Verification items for the finished model (mm, model axes). A direction names the side the tool comes from. Round coordinates to 2 decimals unless told otherwise and drop trailing zeros. Order: outer loops, then holes, each group sorted by start corner. A loop starts at its lowest first (then second) coordinate and runs counter-clockwise, first axis right, second up. Notation, with made-up numbers: M 52,71.5 L 82,71.5 A29 ccw 82,99.5 Z; hole C 33,8 d10. An arc over 180 degrees is marked long. Use one line per item in the form item = value. Start each with the question number.
Item 1: Thickness scan on probe 1 along Z at (x, y) = (-10, -26.5); probe 2 along X at (y, z) = (-9, -8.5); probe 3 along Z at (x, y) = (49.5, -9). Record the ranges inside material, lowest first. Write a range as [from, to].
Item 2: Release check for a two-part mould opening along X. For faces 1 (the cylindrical face through (15.86, -41.49, 1.72)), 2 (the flat face through (17, -41, -49.969)), 3 (the cylindrical face through (16.509, -11.997, -2.13)) record: +X half, -X half, draft (parallel to the pull), parting line (faces both ways), or undercut.
Item 3: Tool access check on faces 4 (the flat face through (20, -29, -28.969)), 5 (the cylindrical face through (15.93, -38.49, -61.98)), 6 (the flat face through (-9.8, -7.8, -15.969)). Record the directions out of +Z, -Z, +X, -X, +Y, -Y that give a thin tool (end or side, any length) a straight path to the whole face; none if there is none.
Item 4: Go/stop test with flat-tipped pins: pin 1 Ø3 at (y, z) = (-30.5, 32.5) entering from -X; pin 2 Ø2 at (y, z) = (-5, -19.5) entering from +X; pin 3 Ø2 at (x, y) = (47, -4) entering from +Z. Record where each tip stops, or that it passes through.
Item 5: Cross-section at A-A on z = 22.5. Enter the section's corners in (x, y).
from build123d import *

# Parameters (mm, degrees)
F2_W      = 103.9337478578
F2_H      = 131.3569024205
F3_DEPTH  = 50
F4_R      = 8
F5_DEPTH  = 7
F6_R      = 7.5
F7_DEPTH  = 2
F8_R      = 6.5
F9_DEPTH  = 11
F10_R     = 3.5
F11_DEPTH = 11
F12_R     = 1.5
F13_DEPTH = 4
F14_R     = 2.5
F15_DEPTH = 15
F17_START = -4
F16_R     = 6.5
F17_DEPTH = 21.001
F19_DEPTH = 3


with BuildPart() as f1:
    # F0 (on Front) → F1 (revolve)
    with BuildSketch(Plane.XZ):
        with BuildLine():
            Line((58.2725809174, 57.0314990246), (54.7725809174, 57.0314990246))
            Line((54.7725809174, 57.0314990246), (54.7725809174, -8.9685009754))
            Line((54.7725809174, -8.9685009754), (33.7725809174, -8.9685009754))
            Line((33.7725809174, -8.9685009754), (33.7725809174, 2.9023842439))
            Line((33.7725809174, 2.9023842439), (30.7725809174, 4.9023842439))
            Line((30.7725809174, 4.9023842439), (28.7725809174, 4.9023842439))
            Line((28.7725809174, 4.9023842439), (28.7725809174, -8.9685009754))
            Line((28.7725809174, -8.9685009754), (26.7725809174, -8.9685009754))
            Line((26.7725809174, -8.9685009754), (26.7725809174, -10.9685009754))
            Line((26.7725809174, -10.9685009754), (26.7725809174, -21.9685009754))
            Line((26.7725809174, -21.9685009754), (16.7725809174, -21.9685009754))
            Line((16.7725809174, -21.9685009754), (16.7725809174, -59.4685009754))
            Line((16.7725809174, -59.4685009754), (53.2725809174, -59.4685009754))
            Line((53.2725809174, -59.4685009754), (53.2725809174, -60.9685009754))
            Line((53.2725809174, -60.9685009754), (55.2725809174, -60.9685009754))
            Line((55.2725809174, -60.9685009754), (55.2725809174, -62.9685009754))
            Line((55.2725809174, -62.9685009754), (53.2725809174, -62.9685009754))
            Line((53.2725809174, -62.9685009754), (53.2725809174, -64.9685009754))
            Line((53.2725809174, -64.9685009754), (58.2725809174, -64.9685009754))
            Line((58.2725809174, -64.9685009754), (58.2725809174, -49.9685009754))
            Line((58.2725809174, -49.9685009754), (56.2725809174, -49.9685009754))
            Line((56.2725809174, -49.9685009754), (56.2725809174, -29.9685009754))
            Line((56.2725809174, -29.9685009754), (58.2725809174, -29.9685009754))
            Line((58.2725809174, -29.9685009754), (58.2725809174, 32.5314990246))
            ThreePointArc((58.2725809174, 32.5314990246), (60.1763868397, 37.1276931023), (64.7725809174, 39.0314990246))
            Line((64.7725809174, 39.0314990246), (64.7725809174, 57.0314990246))
            Line((64.7725809174, 57.0314990246), (58.2725809174, 57.0314990246))
        make_face()
    revolve(axis=Axis((16.7725809174, 0, -11.2093901262), (0, 0, 1)))

    # F2 (on Front) → F3 (cut)
    with BuildSketch(Plane.XZ):
        with Locations((15.4789481312, -5.4226405919)):
            Rectangle(F2_W, F2_H)
    extrude(amount=-F3_DEPTH, mode=Mode.SUBTRACT)

    # F4 (on face) → F5 (cut)
    with BuildSketch(Plane.XY.offset(-8.9685009754)):
        with BuildLine():
            Line((-1.7274190826, 0), (-17.7274190826, 0))
            ThreePointArc((-17.7274190826, 0), (-9.7274190826, -8), (-1.7274190826, 0))
        make_face()
        with BuildLine():
            ThreePointArc((36.2725809174, 0), (44.2725809174, -8), (52.2725809174, 0))
            Line((52.2725809174, 0), (36.2725809174, 0))
        make_face()
        with Locations((16.7725809174, -26.5)):
            Circle(F4_R)
    extrude(amount=-F5_DEPTH, mode=Mode.SUBTRACT)

    # F6 (on face) → F7 (cut)
    with BuildSketch(Plane.XY.offset(-15.9685009754)):
        with BuildLine():
            Line((-2.2274190826, 0), (-17.2274190826, 0))
            ThreePointArc((-17.2274190826, 0), (-9.7274190826, -7.5), (-2.2274190826, 0))
        make_face()
        with BuildLine():
            Line((51.7725809174, 0), (36.7725809174, 0))
            ThreePointArc((36.7725809174, 0), (44.2725809174, -7.5), (51.7725809174, 0))
        make_face()
        with Locations((16.7725809174, -26.5)):
            Circle(F6_R)
    extrude(amount=-F7_DEPTH, mode=Mode.SUBTRACT)

    # F8 (on face) → F9 (cut)
    with BuildSketch(Plane.XY.offset(-17.9685009754)):
        with BuildLine():
            Line((-3.2274190826, 0), (-16.2274190826, 0))
            ThreePointArc((-16.2274190826, 0), (-9.7274190826, -6.5), (-3.2274190826, 0))
        make_face()
        with BuildLine():
            Line((50.7725809174, 0), (37.7725809174, 0))
            ThreePointArc((37.7725809174, 0), (44.2725809174, -6.5), (50.7725809174, 0))
        make_face()
        with Locations((16.7725809174, -26.5)):
            Circle(F8_R)
    extrude(amount=-F9_DEPTH, mode=Mode.SUBTRACT)

    # F10 (on face) → F11 (cut)
    with BuildSketch(Plane.XY.offset(-28.9685009754)):
        with BuildLine():
            Line((-6.2274190826, 0), (-13.2274190826, 0))
            ThreePointArc((-13.2274190826, 0), (-9.7274190826, -3.5), (-6.2274190826, 0))
        make_face()
        with BuildLine():
            Line((47.7725809174, 0), (40.7725809174, 0))
            ThreePointArc((40.7725809174, 0), (44.2725809174, -3.5), (47.7725809174, 0))
        make_face()
        with Locations((16.7725809174, -26.5)):
            Circle(F10_R)
    extrude(amount=-F11_DEPTH, mode=Mode.SUBTRACT)

    # F12 (on face) → F13 (cut)
    with BuildSketch(Plane.XY.offset(-39.9685009754)):
        with Locations((-11.7274190826, 0)):
            Circle(F12_R)
        with BuildLine():
            ThreePointArc((44.7725809174, 0), (46.2725809174, -1.5), (47.7725809174, 0))
            Line((47.7725809174, 0), (44.7725809174, 0))
        make_face()
    extrude(amount=-F13_DEPTH, mode=Mode.SUBTRACT)

    # F14 (on face) → F15 (cut)
    with BuildSketch(Plane.XY.offset(57.0314990246)):
        with BuildLine():
            Line((-23.7274190826, 0), (-28.7274190826, 0))
            ThreePointArc((-28.7274190826, 0), (-26.2274190826, -2.5), (-23.7274190826, 0))
        make_face()
        with Locations((16.7725809174, -43)):
            Circle(F14_R)
        with BuildLine():
            ThreePointArc((57.2725809174, 0), (59.7725809174, -2.5), (62.2725809174, 0))
            Line((62.2725809174, 0), (57.2725809174, 0))
        make_face()
    extrude(amount=-F15_DEPTH, mode=Mode.SUBTRACT)

    # F16 (on face) → F17 (cut)
    with BuildSketch(Plane.XY.offset(-39.9685009754).offset(F17_START)):
        with Locations((44.2725809174, 0)):
            Circle(F16_R)
        with BuildLine():
            ThreePointArc((47.7725809174, 0), (44.2725809174, -3.5), (40.7725809174, 0))
            Line((40.7725809174, 0), (44.7725809174, 0))
            ThreePointArc((44.7725809174, 0), (46.2725809174, -1.5), (47.7725809174, 0))
        make_face(mode=Mode.SUBTRACT)
        with BuildLine():
            Line((44.7725809174, 0), (40.7725809174, 0))
            ThreePointArc((40.7725809174, 0), (44.2725809174, -3.5), (47.7725809174, 0))
            ThreePointArc((47.7725809174, 0), (46.2725809174, -1.5), (44.7725809174, 0))
        make_face()
    extrude(amount=-F17_DEPTH, mode=Mode.SUBTRACT)

    # F18 (on face) → F19 (cut)
    with BuildSketch(Plane(origin=(0, 0, -59.4685009754), x_dir=(1, 0, 0), z_dir=(0, 0, -1))):
        with BuildLine():
            Line((50.7725809174, 0), (52.5225809174, 0))
            ThreePointArc((52.5225809174, 0), (44.2725809174, 8.25), (36.0225809174, 0))
            Line((36.0225809174, 0), (37.7725809174, 0))
            ThreePointArc((37.7725809174, 0), (44.2725809174, 6.5), (50.7725809174, 0))
        make_face()
    extrude(amount=-F19_DEPTH, mode=Mode.SUBTRACT)


solid = f1.part
Output values:
q1.probe_1 = [-64.97, -62.97], [-60.97, -8.97]
q1.probe_2 = [-23.74, -20.15], [2.35, 8.84], [24.71, 31.19], [53.69, 57.28]
q1.probe_3 = [-59.47, -8.97]
q2.face_1 = parting line
q2.face_2 = draft
q2.face_3 = undercut
q3.face_4 = +Z
q3.face_5 = +Y
q3.face_6 = +Z, +Y
q4.pin_1 = -12.91
q4.pin_2 = 58.08
q4.pin_3 = -28.97
q5.outline = M -24.73,0 A41.5 ccw 58.27,0 L 54.77,0 A38 cw -21.23,0 Z
